Input: part model. Units: mm. Frame: model coordinates. A direction names the side the tool comes from. Coordinates: 2 decimals unless noted, no trailing zeros. Order: outer loops, then holes, each group sorted by start corner. A loop starts at its lowest first (then second) coordinate and runs counter-clockwise, first axis right, second up. Notation, with made-up numbers: (-3.5, 59) -> (8.5, 59) arc R22 cw to (8.5, 84) -> close; hole circle Ø1 at (-30.5, -30.75). An arc over 180 degrees is marked (long way). Use one line per item in the form item = value. Start each with the question number.
1) Draft query along Z for faces 5 (the cylindrical face through (-24.24, 2.96, -35.06)), 6 (the flat face through (-31, 4, 23.4)), 7 (the flat face through (-26, 6, 16)). Return one class per face: pulls with the +Z half, pulls with the -Z half, needs draft (parallel to the pull), parting line crosses it, or undercut.
2) Section query D-D on z = -26. Output: boundary loops of the cut face in (x, y), then the cut area to 3 significant figures.
3) Ray query, line 1 along Z through (x, y) = (-8.5, 3.5); line 2 along Z through (x, y) = (-44.5, 0.5); line 3 along X through (y, z) = (5.5, 9). Return the intervals inside material, ascending.
4) Pin query (flat end, axial travel): pin 1 (1.5 mm diameter, centred on x = -21, y = 1.5, fed in from +Z); pin 2 (0.9 mm diameter, centred on x = -33, z = 1.5, fed in from +Y); pin 3 (1.5 mm diameter, centred on x = -22, y = 1.5, fed in from -Z). Return the tip coordinate at first contact, or that it passes through.
5) Access query for faces 1 (the flat face through (-26, 2, -10.6)), 2 (the flat face through (-46.612, 5, -15)), 3 (the flat face through (-26, 0, 16)), 4 (the flat face through (-26, 3, 37)). Directions: +Z, -Z, +X, -X, +Y, -Y. A direction counts if a zero-diameter tool reaches every point of the face in a straight line with its end or side. Return the directions, or none.
6) Section query B-B on z = 11. Output: boundary loops of the cut face in (x, y), then the cut area to 3 significant figures.
7) Section query A-A on x = -33.5. Output: boundary loops of the cut face in (y, z).
8) Section query C-C on x = -62.5. Output: boundary loops of the cut face in (y, z), then the cut area to 3 significant figures.
from build123d import *

# Parameters (mm, degrees)
SKETCH1_R              = 42.5
BOSS_EXTRUDE1_DEPTH    = 6
SKETCH2_W              = 20.5
SKETCH2_H              = 15.5
CUT_EXTRUDE1_DEPTH     = 3
CUT_EXTRUDE2_DEPTH     = 20.5
CUT_EXTRUDE3_REACH     = 86.892
SKETCH4_W              = 41
SKETCH4_H              = 9.5
SKETCH5_R              = 1.5
FILLET1_R              = 1.5
LPATTERN4_COUNT        = 3
LPATTERN4_PITCH        = 23.25
FILLET1_OF_LPATTERN4_R = 1.5


with BuildPart() as part:
    # Sketch1 → Boss-Extrude1 (new body)
    with BuildSketch(Plane(origin=(0, 0, 0), x_dir=(1, 0, 0), z_dir=(0, 1, 0))):
        with Locations(Location((-26.111816808, -7.400353612, 0), (0, 0, 270))):
            Circle(SKETCH1_R)
    extrude(amount=BOSS_EXTRUDE1_DEPTH)

    # Sketch2 → Cut-Extrude1 (cut)
    with BuildSketch(Plane(origin=(0, 6, 0), x_dir=(1, 0, 0), z_dir=(0, 1, 0))):
        with Locations((-36.361816808, 15.349646388)):
            Rectangle(SKETCH2_W, SKETCH2_H)
    cut_extrude1 = extrude(amount=-CUT_EXTRUDE1_DEPTH, mode=Mode.SUBTRACT)

    # Sketch3 → Cut-Extrude2 (cut)
    with BuildSketch(Plane.ZY.offset(26.111816808)):
        Polygon((-23.099646388, 3), (-7.599646388, 3), (-7.599646388, 4.2), (-8.599646388, 4.2), (-8.599646388, 6), (-22.099646388, 6), (-22.099646388, 4.2), (-23.099646388, 4.2), align=None)
    cut_extrude2 = extrude(amount=-CUT_EXTRUDE2_DEPTH, mode=Mode.SUBTRACT)

    # Sketch4 → Cut-Extrude3 (cut, up to next)
    with BuildSketch(Plane(origin=(0, 3, 0), x_dir=(1, 0, 0), z_dir=(0, 1, 0)), mode=Mode.PRIVATE) as cut_extrude3_sk1:
        with Locations((-26.111816808, 15.349646388)):
            Rectangle(SKETCH4_W, SKETCH4_H)
    cut_extrude3_tool1 = extrude(cut_extrude3_sk1.sketch, amount=-CUT_EXTRUDE3_REACH, mode=Mode.PRIVATE) & part.part
    cut_extrude3 = cut_extrude3_tool1.solids().sort_by_distance((-26.111817, 3, -15.349646))[0]
    add(cut_extrude3, mode=Mode.SUBTRACT)

    # Sketch5 → Cut-Revolve1 (revolve, cut)
    with BuildSketch(Plane(origin=(-46.611816808, 0, 0), x_dir=(0, 0, -1), z_dir=(1, 0, 0)), mode=Mode.PRIVATE) as cut_revolve1_sk:
        with Locations((15.348547186, 3)):
            Circle(SKETCH5_R)
    cut_revolve1 = revolve(cut_revolve1_sk.sketch.rotate(Axis((-46.611816808, 6, -23.099646388), (0, 0, 1)), 315), axis=Axis((-46.611816808, 6, -23.099646388), (0, 0, 1)), mode=Mode.SUBTRACT)

    # Fillet1
    fillet1_edges = [part.edges().sort_by_distance(p)[0] for p in [
        (-26.111816808, 4.2, -8.099646388),
        (-26.111816808, 4.2, -22.599646388),
    ]]
    fillet(fillet1_edges, radius=FILLET1_R)

    # LPattern4: Cut-Extrude1, Cut-Extrude2, Cut-Extrude3, Cut-Revolve1 ×3
    with Locations(*[(0, 0, i * LPATTERN4_PITCH) for i in range(1, LPATTERN4_COUNT)]):
        add(cut_extrude1, mode=Mode.SUBTRACT)
        add(cut_extrude2, mode=Mode.SUBTRACT)
        add(cut_extrude3, mode=Mode.SUBTRACT)
        add(cut_revolve1, mode=Mode.SUBTRACT)

    # Fillet1 of LPattern4
    fillet1_of_lpattern4_edges = [part.edges().sort_by_distance(p)[0] for p in [
        (-26.111816808, 4.2, 15.150353612),
        (-26.111816808, 4.2, 0.650353612),
        (-26.111816808, 4.2, 38.400353612),
        (-26.111816808, 4.2, 23.900353612),
    ]]
    fillet(fillet1_of_lpattern4_edges, radius=FILLET1_OF_LPATTERN4_R)


solid = part.part
Answers below:
q1.face_5 = parting line crosses it
q1.face_6 = undercut
q1.face_7 = needs draft
q2.outline = (-52.39, 0) -> (0.17, 0) -> (0.17, 6) -> (-52.39, 6) -> close
q2.area = 315 mm^2
q3.line_1 = -31.28 to -23.1, -7.6 to 0.15, 15.65 to 23.4, 38.9 to 46.08
q3.line_2 = -30.92 to -20.1, -10.6 to 3.15, 12.65 to 26.4, 35.9 to 45.72
q3.line_3 = -68.58 to -50.6, -48.53 to -46.61, -5.61 to 16.36
q4.pin_1 = 49.68
q4.pin_2 = 3
q4.pin_3 = -34.97
q5.face_1 = +Y, -Y
q5.face_2 = +Y
q5.face_3 = +Z, -Z, +X, -X, -Y
q5.face_4 = none
q6.outline = (-68.46, 0) -> (-46.61, 0) -> (-46.61, 6) -> (-68.46, 6) -> close; (-5.61, 0) -> (16.24, 0) -> (16.24, 6) -> (-5.61, 6) -> close
q6.area = 262 mm^2
q7.outline = (0, -34.45) -> (6, -34.45) -> (6, -23.1) -> (3, -23.1) -> (3, -20.1) -> (0, -20.1) -> close; (0, -10.6) -> (3, -10.6) -> (3, -7.6) -> (6, -7.6) -> (6, 0.15) -> (3, 0.15) -> (3, 3.15) -> (0, 3.15) -> close; (0, 12.65) -> (3, 12.65) -> (3, 15.65) -> (6, 15.65) -> (6, 23.4) -> (3, 23.4) -> (3, 26.4) -> (0, 26.4) -> close; (0, 35.9) -> (3, 35.9) -> (3, 38.9) -> (6, 38.9) -> (6, 49.25) -> (0, 49.25) -> close
q8.outline = (0, -14.56) -> (6, -14.56) -> (6, 29.36) -> (0, 29.36) -> close
q8.area = 263 mm^2
